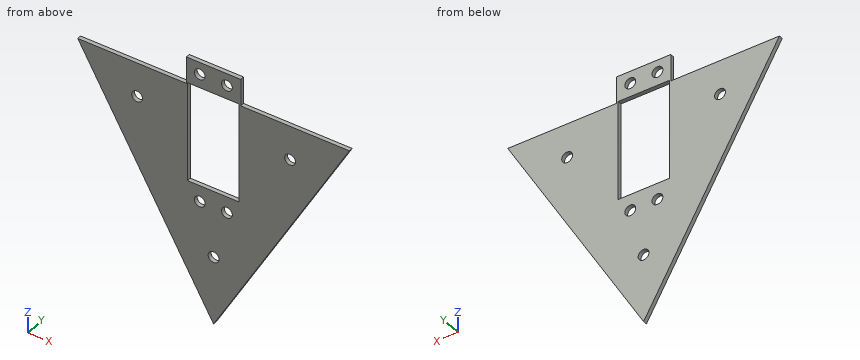
from build123d import *

# Parameters (mm, degrees)
BASE_FLANGE1_DEPTH = 1.5
SKETCH6_R          = 2
CUT_EXTRUDE1_DEPTH = 10
SKETCH7_R          = 2
SKETCH7_W          = 19
SKETCH7_H          = 37
CUT_EXTRUDE2_DEPTH = 10


# Sheet-metal steps are written as plain solids
with BuildPart() as part:
    # Sketch1 → Base-Flange1 (new body)
    with BuildSketch(Plane(origin=(0, 0, 0), x_dir=(1, 0, 0), z_dir=(0, 1, 0))):
        Polygon((0, 57.735026919), (-50, -28.867513459), (-10, -28.867513459), (-10, -38.867513459), (10, -38.867513459), (10, -28.867513459), (50, -28.867513459), align=None)
    extrude(amount=-BASE_FLANGE1_DEPTH)

    # Sketch6 → Cut-Extrude1 (cut)
    with BuildSketch(Plane(origin=(0, 0, 0), x_dir=(1, 0, 0), z_dir=(0, 1, 0))):
        with Locations(Location((0, 32.5, 0), (0, 0, 270))):
            Circle(SKETCH6_R)
        with Locations(Location((28.145825623, -16.25, 0), (0, 0, 270))):
            Circle(SKETCH6_R)
        with Locations(Location((-28.145825623, -16.25, 0), (0, 0, 270))):
            Circle(SKETCH6_R)
    extrude(amount=-CUT_EXTRUDE1_DEPTH, mode=Mode.SUBTRACT)

    # Sketch7 → Cut-Extrude2 (cut)
    with BuildSketch(Plane(origin=(0, 0, 0), x_dir=(1, 0, 0), z_dir=(0, 1, 0))):
        with Locations(Location((-5.1, -34.347513459, 0), (0, 0, 270))):
            Circle(SKETCH7_R)
        with Locations(Location((4.9, -34.347513459, 0), (0, 0, 270))):
            Circle(SKETCH7_R)
        with Locations(Location((-5.1, 13.652486541, 0), (0, 0, 270))):
            Circle(SKETCH7_R)
        with Locations(Location((4.9, 13.652486541, 0), (0, 0, 270))):
            Circle(SKETCH7_R)
        with Locations((-0.1, -10.827513459)):
            Rectangle(SKETCH7_W, SKETCH7_H)
    extrude(amount=-CUT_EXTRUDE2_DEPTH, mode=Mode.SUBTRACT)


solid = part.part
Geometry check sheet. Reference: the model listing, model coordinates, mm. Coordinates: 2 decimals unless noted, no trailing zeros. Order: outer loops, then holes, each group sorted by start corner. A loop starts at its lowest first (then second) coordinate and runs counter-clockwise, first axis right, second up. Notation, with made-up numbers: (3.25, -28.5) - (32.25, -28.5) arc R6 ccw to (32.25, -18.5) - close; hole circle Ø5 at (57.25, 36). An arc over 180 degrees is marked (long way). Answer in a Markdown table with one row per item. Add a question column.
1) Material ranges on line 1 along X through (y, z) = (-0.1, 20); line 2 along Z through (x, y) = (-6, -1.3); line 3 along X through (y, z) = (-0.15, 6), recorded low to high. Write a range as [from, to].
2) Cross-section at A-A, the plane z = -33. Record the cut outline in (x, y).
3) Cross-section at B-B, the plane x = 4.9. Record the cut outline in (y, z), then the cut area to 3 significant figures.
4) Gauge pin test, flat ends, axial feed: P1, Ø3.5, axis at x = 0, z = -32.5, coming from the -Y side; P2, Ø0.8, axis at y = -0.5, z = 34.5, coming from the +X side; P3, Ø0.8, axis at x = -4, y = -1, coming from the -Z side; P4, Ø0.8, axis at y = -1, z = 5, coming from the +X side. Record the tip position at first contact, or that the pin passes through.
5) Cross-section at D-D, the plane z = 16.25. Record the cut outline in (x, y), then the cut area to 3 significant figures.
6) Cross-section at C-C, the plane y = -0.45. State how many separate pieces and enclosed holes the cut face has, then the cut area to 3 significant figures.
Check result:
| question | item | result |
|---|---|---|
| 1 | line 1 | x = [-44.88, -9.6], [9.4, 44.88] |
| 1 | line 2 | z = [-47.34, -15.44], [-11.87, -7.67], [29.33, 32.56], [36.13, 38.87] |
| 1 | line 3 | x = [-36.8, -9.6], [9.4, 36.8] |
| 2 | outline | (-14.28, -1.5) - (-1.94, -1.5) - (-1.94, 0) - (-14.28, 0) - close; (1.94, -1.5) - (14.28, -1.5) - (14.28, 0) - (1.94, 0) - close |
| 3 | outline | (-1.5, -49.25) - (0, -49.25) - (0, -15.65) - (-1.5, -15.65) - close; (-1.5, -11.65) - (0, -11.65) - (0, -7.67) - (-1.5, -7.67) - close; (-1.5, 29.33) - (0, 29.33) - (0, 32.35) - (-1.5, 32.35) - close; (-1.5, 36.35) - (0, 36.35) - (0, 38.87) - (-1.5, 38.87) - close |
| 3 | area | 64.7 mm² |
| 4 | P1 | passes through |
| 4 | P2 | stops at x = 10 |
| 4 | P3 | stops at z = -51.5 |
| 4 | P4 | stops at x = 36.45 |
| 5 | outline | (-42.72, -1.5) - (-30.15, -1.5) - (-30.15, 0) - (-42.72, 0) - close; (-26.15, -1.5) - (-9.6, -1.5) - (-9.6, 0) - (-26.15, 0) - close; (9.4, -1.5) - (26.15, -1.5) - (26.15, 0) - (9.4, 0) - close; (30.15, -1.5) - (42.72, -1.5) - (42.72, 0) - (30.15, 0) - close |
| 5 | area | 87.6 mm² |
| 6 | separate pieces | 1 |
| 6 | enclosed holes | 8 |
| 6 | area | 3,740 mm² |
